Verification items for the finished model (mm, model axes). A direction names the side the tool comes from. Give positions to 0.01 mm unless a question says otherwise; leave off trailing zeros. Loops run counter-clockwise (first coordinate to the right, second up) from the corner with the lowest first, then second, coordinate; pieces in that order, holes last. Notation, with made-up numbers: (1, 63) - (17, 63) arc R19 cw to (17, 70) - close; hole circle Ø10 at (81, 58). An arc over 180 degrees is marked (long way). One line per item, written item: value. Start each with the question number.
1. Sectioned sample at A-A (y = 0). Record the cut outline in (x, z), plus the area to 3 significant figures.
2. Sectioned sample at D-D (x = 53.5). Record the cut outline in (y, z), plus the area to 3 significant figures.
3. Sectioned sample at B-B (z = 0). Record the cut outline in (x, y), plus the area to 3 significant figures.
4. Scan lines: L1, parallel to Y at x = 55, z = 0; L2, parallel to Z at x = 68.5, y = -1.25; L3, parallel to Z at x = 67, y = 3.75. Record each from-to range of solid material in increasing order. Write a range as [from, to].
5. Access from +Z, -Z, +X, -X, +Y, -Y to the whole of each face (thin tool, end or side, straight path). Record for faces 4 (the flat face through (0, 9, -5)), 5 (the cylindrical face through (63.25, -0.07, -10.24)).
6. Gauge pin test, flat ends, axial feed: pin 1 (1.5 mm diameter, centred on x = 27.5, y = -7.5, fed in from -Z); pin 2 (10 mm diameter, centred on x = 61, y = -8.5, fed in from -Z); pin 3 (4 mm diameter, centred on x = 52, y = -5.5, fed in from +Z); pin 4 (6.5 mm diameter, centred on y = 0.5, z = 5, fed in from +X). Record the tip position at first contact, or that the pin passes through.
7. Sectioned sample at C-C (y = 4.5). Record the cut outline in (x, z), plus the area to 3 significant figures.
8. Mould release check, pull along X, two halves, no side actions. Record for faces 1 (the cylindrical face through (35.66, -1.4, 10.66)), 2 (the flat face through (72, 9, -5)), 3 (the flat face through (0, -9, -5)): pulls with the +X half, pulls with the -X half, needs draft (parallel to the pull), parting line crosses it, or undercut.
from build123d import *

# Parameters (mm, degrees)
F0_R      = 11
F1_DEPTH  = 12
F2_R      = 10.75
F3_DEPTH  = 48
F4_R      = 11
F4_R_2    = 10.75
F5_DEPTH  = 12
F7_D      = 20
F9_DEPTH  = 10
F11_DEPTH = 10
F14_DEPTH = 5


with BuildPart() as f1:
    # F0 (on Right) → F1 (new body)
    with BuildSketch(Plane.YZ):
        Circle(F0_R)
    extrude(amount=F1_DEPTH)

    # F2 (on face) → F3 (join)
    with BuildSketch(Plane.YZ.offset(12)):
        Circle(F2_R)
    extrude(amount=F3_DEPTH)

    # F4 (on face) → F5 (join)
    with BuildSketch(Plane.YZ.offset(60)):
        Circle(F4_R)
        Circle(F4_R_2, mode=Mode.SUBTRACT)
        Circle(F4_R_2)
    extrude(amount=F5_DEPTH)

    # F7 (through all)
    with Locations(Plane(origin=(0, 0, 0), x_dir=(0, -1, 0), z_dir=(-1, 0, 0))):
        with Locations((0, 0)):
            Hole(F7_D / 2)

    # F8 (on face) → F9 (cut)
    with BuildSketch(Plane(origin=(0, 0, 0), x_dir=(0, -1, 0), z_dir=(-1, 0, 0))):
        with BuildLine():
            Line((1.6634346337, 10.8734992169), (1.5748160855, 10.370918456))
            Line((1.5748160855, 10.370918456), (1.489737103, 9.8884115693))
            ThreePointArc((1.489737103, 9.8884115693), (1.7407460416, 9.8473246732), (1.9906288286, 9.7998671862))
            Line((1.9906288286, 9.7998671862), (2.1643298383, 10.7849745642))
            ThreePointArc((2.1643298383, 10.7849745642), (1.9143939946, 10.8321325524), (1.6634346337, 10.8734992169))
        make_face()
        with BuildLine():
            ThreePointArc((-1.9821409796, 9.8015874805), (-1.7364817767, 9.8480775301), (-1.489737103, 9.8884115693))
            Line((-1.489737103, 9.8884115693), (-1.572378121, 10.3570920718))
            Line((-1.572378121, 10.3570920718), (-1.6634346337, 10.8734992169))
            ThreePointArc((-1.6634346337, 10.8734992169), (-1.9101299543, 10.8328852831), (-2.1558385102, 10.786675128))
            Line((-2.1558385102, 10.786675128), (-2.0647819975, 10.270267983))
            Line((-2.0647819975, 10.270267983), (-1.9821409796, 9.8015874805))
        make_face()
        with BuildLine():
            Line((9.9267039757, -3.3469803284), (9.4794942453, -3.1842092981))
            ThreePointArc((9.4794942453, -3.1842092981), (9.3969262079, -3.4202014333), (9.3084841736, -3.6540556085))
            Line((9.3084841736, -3.6540556085), (9.755693904, -3.8168266388))
            Line((9.755693904, -3.8168266388), (10.2484438667, -3.9961729581))
            ThreePointArc((10.2484438667, -3.9961729581), (10.3366188286, -3.7622215766), (10.4194539383, -3.5263266477))
            Line((10.4194539383, -3.5263266477), (9.9267039757, -3.3469803284))
        make_face()
        with BuildLine():
            ThreePointArc((-9.3084841736, -3.6540556085), (-9.3984063471, -3.416132043), (-9.4822483512, -3.175998458))
            Line((-9.4822483512, -3.175998458), (-10.4222268709, -3.51812266))
            ThreePointArc((-10.4222268709, -3.51812266), (-10.3380989649, -3.758152444), (-10.2484438667, -3.9961729581))
            Line((-10.2484438667, -3.9961729581), (-9.7688868862, -3.8216284916))
            Line((-9.7688868862, -3.8216284916), (-9.3084841736, -3.6540556085))
        make_face()
        with BuildLine():
            Line((8.1940708007, -6.5492899644), (7.8187470706, -6.2343559608))
            ThreePointArc((7.8187470706, -6.2343559608), (7.6576603054, -6.4311926302), (7.4916195226, -6.6238687282))
            Line((7.4916195226, -6.6238687282), (8.2578970327, -7.2668519042))
            ThreePointArc((8.2578970327, -7.2668519042), (8.4237049702, -7.0739801084), (8.585009233, -6.8773262587))
            Line((8.585009233, -6.8773262587), (8.1940708007, -6.5492899644))
        make_face()
        with BuildLine():
            ThreePointArc((-7.4973532657, -6.6173781824), (-7.6604444312, -6.4278760969), (-7.8187470706, -6.2343559608))
            Line((-7.8187470706, -6.2343559608), (-8.1833157831, -6.540265433))
            Line((-8.1833157831, -6.540265433), (-8.585009233, -6.8773262587))
            ThreePointArc((-8.585009233, -6.8773262587), (-8.4264888743, -7.0706637066), (-8.2636154282, -7.2603484803))
            Line((-8.2636154282, -7.2603484803), (-7.8619219782, -6.9232876546))
            Line((-7.8619219782, -6.9232876546), (-7.4973532657, -6.6173781824))
        make_face()
    extrude(amount=-F9_DEPTH, mode=Mode.SUBTRACT)

    # F10 (on face) → F11 (cut)
    with BuildSketch(Plane.YZ.offset(72)):
        with BuildLine():
            ThreePointArc((-1.9821409796, 9.8015874805), (-1.7364817767, 9.8480775301), (-1.489737103, 9.8884115693))
            Line((-1.489737103, 9.8884115693), (-1.6634346337, 10.8734992169))
            ThreePointArc((-1.6634346337, 10.8734992169), (-1.9101299543, 10.8328852831), (-2.1558385102, 10.786675128))
            Line((-2.1558385102, 10.786675128), (-1.9821409796, 9.8015874805))
        make_face()
        with BuildLine():
            Line((1.6634346337, 10.8734992169), (1.489737103, 9.8884115693))
            ThreePointArc((1.489737103, 9.8884115693), (1.7364817767, 9.8480775301), (1.9821409796, 9.8015874805))
            Line((1.9821409796, 9.8015874805), (2.1558385102, 10.786675128))
            ThreePointArc((2.1558385102, 10.786675128), (1.9101299543, 10.8328852831), (1.6634346337, 10.8734992169))
        make_face()
        with BuildLine():
            Line((10.4194539383, -3.5263266477), (9.4794942453, -3.1842092981))
            ThreePointArc((9.4794942453, -3.1842092981), (9.3969262079, -3.4202014333), (9.3084841736, -3.6540556085))
            Line((9.3084841736, -3.6540556085), (10.2484438667, -3.9961729581))
            ThreePointArc((10.2484438667, -3.9961729581), (10.3366188286, -3.7622215766), (10.4194539383, -3.5263266477))
        make_face()
        with BuildLine():
            Line((8.585009233, -6.8773262587), (7.8187470706, -6.2343559608))
            ThreePointArc((7.8187470706, -6.2343559608), (7.6604444312, -6.4278760969), (7.4973532657, -6.6173781824))
            Line((7.4973532657, -6.6173781824), (8.2636154282, -7.2603484803))
            ThreePointArc((8.2636154282, -7.2603484803), (8.4264888743, -7.0706637066), (8.585009233, -6.8773262587))
        make_face()
        with BuildLine():
            ThreePointArc((-9.3084841736, -3.6540556085), (-9.3969262079, -3.4202014333), (-9.4794942453, -3.1842092981))
            Line((-9.4794942453, -3.1842092981), (-10.4194539383, -3.5263266477))
            ThreePointArc((-10.4194539383, -3.5263266477), (-10.3366188286, -3.7622215766), (-10.2484438667, -3.9961729581))
            Line((-10.2484438667, -3.9961729581), (-9.3084841736, -3.6540556085))
        make_face()
        with BuildLine():
            ThreePointArc((-7.4973532657, -6.6173781824), (-7.6604444312, -6.4278760969), (-7.8187470706, -6.2343559608))
            Line((-7.8187470706, -6.2343559608), (-8.585009233, -6.8773262587))
            ThreePointArc((-8.585009233, -6.8773262587), (-8.4264888743, -7.0706637066), (-8.2636154282, -7.2603484803))
            Line((-8.2636154282, -7.2603484803), (-7.4973532657, -6.6173781824))
        make_face()
    extrude(amount=-F11_DEPTH, mode=Mode.SUBTRACT)

    # F13 (on offset) → F14 (cut)
    with BuildSketch(Plane.XY.offset(-11)):
        with BuildLine():
            Line((24, -3.25), (60, -3.25))
            ThreePointArc((60, -3.25), (63.25, 0), (60, 3.25))
            Line((60, 3.25), (24, 3.25))
            ThreePointArc((24, 3.25), (20.75, 0), (24, -3.25))
        make_face()
    extrude(amount=F14_DEPTH, mode=Mode.SUBTRACT)


solid = f1.part
Results are:
1. outline: (0, -11) - (12, -11) - (12, -10.75) - (20.75, -10.75) - (20.75, -10) - (0, -10) - close; (0, 10) - (72, 10) - (72, 11) - (60, 11) - (60, 10.75) - (12, 10.75) - (12, 11) - (0, 11) - close; (63.25, -11) - (72, -11) - (72, -10) - (63.25, -10) - close
1. area: 87.3 mm^2
2. outline: (-3.25, -10.25) - (-3.25, -9.46) arc R10 cw (long way) to (3.25, -9.46) - (3.25, -10.25) arc R10.75 ccw (long way) to start
2. area: 43.9 mm^2
3. outline: (0, -11) - (12, -11) - (12, -10.75) - (60, -10.75) - (60, -11) - (72, -11) - (72, -10) - (0, -10) - close; (0, 10) - (72, 10) - (72, 11) - (60, 11) - (60, 10.75) - (12, 10.75) - (12, 11) - (0, 11) - close
3. area: 120 mm^2
4. L1: y = [-10.75, -10], [10, 10.75]
4. L2: z = [-10.93, -9.92], [9.92, 10.93]
4. L3: z = [-10.34, -9.27], [9.27, 10.34]
5. face 4: +Z, -Z, -X, +Y, -Y
5. face 5: -Z
6. pin 1: stops at z = -8.37
6. pin 2: stops at z = -10.43
6. pin 3: stops at z = 10.16
6. pin 4: passes through
7. outline: (0, -10.04) - (12, -10.04) - (12, -9.76) - (60, -9.76) - (60, -10.04) - (72, -10.04) - (72, -8.93) - (0, -8.93) - close; (0, 8.93) - (72, 8.93) - (72, 10.04) - (60, 10.04) - (60, 9.76) - (12, 9.76) - (12, 10.04) - (0, 10.04) - close
7. area: 133 mm^2
8. face 1: undercut
8. face 2: pulls with the +X half
8. face 3: pulls with the -X half
